Source: CAD feature listing. Evaluate the final solid. Frame: model axes, mm. A direction names the side the tool comes from. Coordinates: 2 decimals unless noted, no trailing zeros. Write each loop counter-clockwise with the first axis right and the second up, starting at its lowest first coordinate (ties: lowest second). Pieces come first, ordered by that corner, then holes. Notation, with made-up numbers: (-14, -4.5) - (19, -4.5) arc R8 ccw to (19, 3.5) - close; hole circle Ø4 at (57.5, -3). An arc over 180 degrees is marked (long way). One line per question, with ' | ' between items.
from build123d import *

# Parameters (mm, degrees)
SKETCH_1_W          = 33.333333334
SKETCH_1_H          = 33.333333334
EXTRUDE_1_DEPTH     = 1.5
SKETCH_2_R          = 3
EXTRUDE_2_DEPTH     = 6
CUT_EXTRUDE_1_DEPTH = 6


with BuildPart() as part:
    # 草图1 → 凸台-拉伸1 (new body)
    with BuildSketch(Plane(origin=(0, 0, 0), x_dir=(1, 0, 0), z_dir=(0, 1, 0))):
        Rectangle(SKETCH_1_W, SKETCH_1_H)
    extrude(amount=EXTRUDE_1_DEPTH)

    # 草图2 → 凸台-拉伸2 (add)
    with BuildSketch(Plane(origin=(0, 1.5, 0), x_dir=(1, 0, 0), z_dir=(0, 1, 0))):
        with Locations(Location((0, 0, 0), (0, 0, 270))):
            Circle(SKETCH_2_R)
    extrude(amount=EXTRUDE_2_DEPTH)

    # 草图3 → 切除-拉伸1 (cut)
    with BuildSketch(Plane(origin=(0, 7.5, 0), x_dir=(1, 0, 0), z_dir=(0, 1, 0))):
        with BuildLine():
            Line((-1.118033989, 1), (1.118033989, 1))
            ThreePointArc((1.118033989, 1), (0, -1.5), (-1.118033989, 1))
        make_face()
    extrude(amount=-CUT_EXTRUDE_1_DEPTH, mode=Mode.SUBTRACT)


solid = part.part
Item 1: Pin query (flat end, axial travel): pin 1 Ø3 at (x, y) = (0, 5.5) entering from +Z; pin 2 Ø5 at (x, z) = (-3, 8.5) entering from -Y; pin 3 Ø0.8 at (x, z) = (0.5, 0.5) entering from +Y. Return the tip coordinate at first contact, or that it passes through.
Check sheet entries:
pin 1: z = 3 | pin 2: y = 0 | pin 3: y = 1.5
Item 2: Cut plane B-B on z = 0. Return loops of the section in (x, y).
Check sheet entries:
outline: (-16.67, 0) - (16.67, 0) - (16.67, 1.5) - (3, 1.5) - (3, 7.5) - (1.5, 7.5) - (1.5, 1.5) - (-1.5, 1.5) - (-1.5, 7.5) - (-3, 7.5) - (-3, 1.5) - (-16.67, 1.5) - close
Item 3: Cut plane C-C on y = 3.25. Return loops of the section in (x, z), and give its area (3 significant figures).
Check sheet entries:
outline: circle Ø6 at (0, 0); hole (-1.12, -1) - (1.12, -1) arc R1.5 ccw (long way) to start | area: 22.0 mm²
Item 4: Cut plane A-A on x = 0. Return loops of the section in (y, z), and give its area (3 significant figures).
Check sheet entries:
outline: (0, -16.67) - (1.5, -16.67) - (1.5, -3) - (7.5, -3) - (7.5, -1) - (1.5, -1) - (1.5, 1.5) - (7.5, 1.5) - (7.5, 3) - (1.5, 3) - (1.5, 16.67) - (0, 16.67) - close | area: 71.0 mm²
Item 5: Ray query, line 1 along X through (y, z) = (5.8, 0); line 2 along Y through (x, z) = (-7, 6); line 3 along X through (y, z) = (3, 1). Return the intervals inside material, ascending. Write a range as [from, to].
Check sheet entries:
line 1: [-3, -1.5], [1.5, 3] | line 2: [0, 1.5] | line 3: [-2.83, -1.12], [1.12, 2.83]
Item 6: Cut plane D-D on x = -13. Return loops of the section in (y, z).
Check sheet entries:
outline: (0, -16.67) - (1.5, -16.67) - (1.5, 16.67) - (0, 16.67) - close
Item 7: Access query for faces 1 (the face through (0, 4.5, 1.5)), 2 (the face through (0, 0, 0)). Directions: +Z, -Z, +X, -X, +Y, -Y. A direction counts if a zero-diameter tool reaches every point of the face in a straight line with its end or side. Return the directions, or none.
Check sheet entries:
face 1: +Y | face 2: +Z, -Z, +X, -X, -Y
Item 8: Mould query, pull axis X, two halves, no side actions, for faces 3 (the face through (0, 5, -1)), 4 (the face through (-16.667, 1, 0)), 5 (the face through (0, 1, -16.667)), 6 (the face through (0, 1.5, 0)). Classes: pulls with the +X half, pulls with the -X half, needs draft (parallel to the pull), parting line crosses it, or undercut.
Check sheet entries:
face 3: undercut | face 4: pulls with the -X half | face 5: needs draft | face 6: undercut
